Source: CAD feature listing. Evaluate the final solid. Frame: model axes, mm. Give positions to 0.01 mm unless a question says otherwise; leave off trailing zeros. Order: outer loops, then holes, each group sorted by start corner. A loop starts at its lowest first (then second) coordinate and runs counter-clockwise, first axis right, second up. Notation, with made-up numbers: M -34.5,59 L 2.5,59 A23 cw 2.5,78 Z; hole C -26.5,-14 d7. An arc over 180 degrees is marked long. Answer as a JSON object with one key per item and string values. Group by question number.
1. Section query B-B (z = 4.3). Output: boundary loops of the cut face in (x, y), plus the area to 3 significant figures.
2. Section query A-A (x = 4.5). Output: boundary loops of the cut face in (y, z), plus the area to 3 significant figures.
3. Material intervals for L1, parallel to Y at x = -8, z = 4.75; L2, parallel to X at y = -0.75, z = 3.2; L3, parallel to Y at x = 4, z = 2.4, sorted ascending. Write a range as [from, to].
4. Pull-direction query (X, two-part tool) for faces 1 (the flat face through (-3, 2, 0)), 2 (the cylindrical face through (-11.39, 8.43, 2.46)), 3 (the cylindrical face through (-5.55, 0.07, 2.46)); classes: +X half, -X half, draft (parallel to the pull), parting line (faces both ways), or undercut.
5. Section query C-C (y = 5.25). Output: boundary loops of the cut face in (x, z), plus the area to 3 significant figures.
6. Section query D-D (x = -1.5). Output: boundary loops of the cut face in (y, z).
from build123d import *

# Parameters (mm, degrees)
SKETCH1_R           = 1.55
SKETCH1_R_2         = 1.7
BOSS_EXTRUDE1_DEPTH = 5


with BuildPart() as part:
    # Sketch1 → Boss-Extrude1 (new body)
    with BuildSketch(Plane.XY):
        with BuildLine():
            Line((-7, -3), (7, -3))
            Line((7, -3), (7, 3))
            Line((7, 3), (-9.5, 9.2))
            ThreePointArc((-9.5, 9.2), (-11.409188309, 8.409188309), (-12.2, 6.5))
            Line((-12.2, 6.5), (-7, -3))
        make_face()
        with Locations((4, 0)):
            Circle(SKETCH1_R, mode=Mode.SUBTRACT)
        with Locations((-4, 0)):
            Circle(SKETCH1_R, mode=Mode.SUBTRACT)
        with Locations((-9.5, 6.5)):
            Circle(SKETCH1_R_2, mode=Mode.SUBTRACT)
    extrude(amount=BOSS_EXTRUDE1_DEPTH)


solid = part.part
Answer sheet:
{
 "1": {"outline": "M -12.2,6.5 L -7,-3 L 7,-3 L 7,3 L -9.5,9.2 A2.7 ccw Z; hole C -9.5,6.5 d3.4; hole C -4,0 d3.1; hole C 4,0 d3.1", "area": "133 mm^2"},
 "2": {"outline": "M -3,0 L -1.47,0 L -1.47,5 L -3,5 Z; M 1.47,0 L 3.94,0 L 3.94,5 L 1.47,5 Z", "area": "20.0 mm^2"},
 "3": {"L1": "[-1.17, 5.7], [7.3, 8.64]", "L2": "[-8.23, -5.36], [-2.64, 2.64], [5.36, 7]", "L3": "[-3, -1.55], [1.55, 4.13]"},
 "4": {"face 1": "draft", "face 2": "-X half", "face 3": "undercut"},
 "5": {"outline": "M -11.52,0 L -10.65,0 L -10.65,5 L -11.52,5 Z; M -8.35,0 L 1.01,0 L 1.01,5 L -8.35,5 Z", "area": "51.1 mm^2"},
 "6": {"outline": "M -3,0 L 6.19,0 L 6.19,5 L -3,5 Z"}
}
